Verification items for the finished model (mm, model axes). A direction names the side the tool comes from. Give positions to 0.01 mm unless a question says otherwise; leave off trailing zeros. Loops run counter-clockwise (first coordinate to the right, second up) from the corner with the lowest first, then second, coordinate; pieces in that order, holes last. Notation, with made-up numbers: (26, 42) - (43, 42) arc R17 ccw to (43, 66) - close; hole circle Ø8 at (-5, -22.5). An arc over 180 degrees is marked (long way). Use one line per item in the form item = value.
```python
from build123d import *

# Parameters (mm, degrees)
CROQUIS1_R              = 47.5
SALIENTE_EXTRUIR1_DEPTH = 9
CROQUIS2_R              = 36
SALIENTE_EXTRUIR2_DEPTH = 22
CROQUIS3_R              = 35.5
SALIENTE_EXTRUIR3_DEPTH = 6
CROQUIS4_R              = 35
SALIENTE_EXTRUIR4_DEPTH = 4
CROQUIS5_R              = 34.5
SALIENTE_EXTRUIR5_DEPTH = 4
CROQUIS6_R              = 34
SALIENTE_EXTRUIR6_DEPTH = 24
REDONDEO1_R             = 5
CHAFL_N1_SIZE           = 5.093697795
CHAFL_N1_SIZE_2         = 12
CORTAR_EXTRUIR1_START   = -59.7
CORTAR_EXTRUIR1_DEPTH   = 59.7
MATRIZC1_COUNT          = 8
SALIENTE_EXTRUIR7_REACH = 91.87
CROQUIS8_W              = 0.328373722
CROQUIS8_H              = 2.57874632


with BuildPart() as part:
    # Croquis1 → Saliente-Extruir1 (new body)
    with BuildSketch(Plane.XY):
        Circle(CROQUIS1_R)
    extrude(amount=SALIENTE_EXTRUIR1_DEPTH)

    # Croquis2 → Saliente-Extruir2 (add)
    with BuildSketch(Plane.XY.offset(9)):
        Circle(CROQUIS2_R)
    extrude(amount=SALIENTE_EXTRUIR2_DEPTH)

    # Croquis3 → Saliente-Extruir3 (add)
    with BuildSketch(Plane.XY.offset(31)):
        Circle(CROQUIS3_R)
    extrude(amount=SALIENTE_EXTRUIR3_DEPTH)

    # Croquis4 → Saliente-Extruir4 (add)
    with BuildSketch(Plane.XY.offset(37)):
        Circle(CROQUIS4_R)
    extrude(amount=SALIENTE_EXTRUIR4_DEPTH)

    # Croquis5 → Saliente-Extruir5 (add)
    with BuildSketch(Plane.XY.offset(41)):
        Circle(CROQUIS5_R)
    extrude(amount=SALIENTE_EXTRUIR5_DEPTH)

    # Croquis6 → Saliente-Extruir6 (add)
    with BuildSketch(Plane.XY.offset(45)):
        Circle(CROQUIS6_R)
    extrude(amount=SALIENTE_EXTRUIR6_DEPTH)

    # Redondeo1
    redondeo1_edges = [part.edges().sort_by_distance(p)[0] for p in [
        (-34, 0, 69),
    ]]
    fillet(redondeo1_edges, radius=REDONDEO1_R)

    # Chaflán1
    # the kernel refuses this chamfer: 12, 5.093697795 mm, written as the material it adds along each edge
    with BuildSketch(Plane(origin=(0, 0, 9), x_dir=(1, 0, 0), z_dir=(0, -1, 0))) as chafl_n1_piece_1_section:
        Polygon((36, CHAFL_N1_SIZE), (36 + CHAFL_N1_SIZE_2, 0), (36, 0), align=None)
    chafl_n1_piece_1 = revolve(axis=Axis((0, 0, 9), (0, 0, 1)), mode=Mode.PRIVATE)
    chafl_n1_piece_1 = chafl_n1_piece_1 & Plane(origin=(0, 0, 11.556485036), x_dir=(1, 0, 0), z_dir=(0, 0, -1)) * Cylinder(47.5, 192, mode=Mode.PRIVATE)
    add(chafl_n1_piece_1)

    # Croquis7 → Cortar-Extruir1 (cut)
    with BuildSketch(Plane.XY.offset(69).offset(CORTAR_EXTRUIR1_START)):
        with BuildLine():
            Line((-47.405168495, 3), (-35.624047548, 3))
            ThreePointArc((-35.624047548, 3), (-35.750143548, 0), (-35.624047548, -3))
            Line((-35.624047548, -3), (-47.405168495, -3))
            ThreePointArc((-47.405168495, -3), (-47.5, 0), (-47.405168495, 3))
        make_face()
    cortar_extruir1 = extrude(amount=CORTAR_EXTRUIR1_DEPTH, mode=Mode.SUBTRACT)

    # MatrizC1: Cortar-Extruir1 ×8 about axis
    matrizc1_axis = Axis((0, 0, 0), (0, 0, 1))
    for i in range(1, MATRIZC1_COUNT):
        add(cortar_extruir1.rotate(matrizc1_axis, i * 360 / MATRIZC1_COUNT), mode=Mode.SUBTRACT)

    # Saliente-Extruir7: up to this face of the body (flat: up to its plane)
    saliente_extruir7_end = Plane(part.part.faces().sort_by_distance((0, 0, 0))[0])
    # Croquis8 → Saliente-Extruir7 (add, up to the picked face)
    with BuildSketch(Plane.XY.offset(9.3), mode=Mode.PRIVATE) as saliente_extruir7_sk1:
        with Locations((47.5, 0)):
            Rectangle(CROQUIS8_W, CROQUIS8_H)
    saliente_extruir7_tool1 = split(extrude(saliente_extruir7_sk1.sketch, amount=-SALIENTE_EXTRUIR7_REACH, mode=Mode.PRIVATE), bisect_by=saliente_extruir7_end, keep=Keep.BOTH, mode=Mode.PRIVATE)
    add(saliente_extruir7_tool1.solids().sort_by(Axis((47.5, 0, 9.3), (0, 0, -1)))[0])


solid = part.part
```
1. Section check B-B, the plane x = 0. Record the cut outline in (y, z), then the cut area to 3 significant figures.
Result set:
outline = (-47.5, 0) - (47.5, 0) - (47.5, 9.21) - (47.29, 9.3) - (35.75, 9.3) - (35.75, 31) - (35.5, 31) - (35.5, 37) - (35, 37) - (35, 41) - (34.5, 41) - (34.5, 45) - (34, 45) - (34, 64) arc R5 ccw to (29, 69) - (-29, 69) arc R5 ccw to (-34, 64) - (-34, 45) - (-34.5, 45) - (-34.5, 41) - (-35, 41) - (-35, 37) - (-35.5, 37) - (-35.5, 31) - (-35.75, 31) - (-35.75, 9.3) - (-47.29, 9.3) - (-47.5, 9.21) - close
area = 5,040 mm²
2. Draft check along X on faces 1 (the cylindrical face through (-35.75, 0.04, 20)), 2 (the flat face through (29.26, -25.02, 12.87)), 3 (the flat face through (-41, 0, 9.3)). Enter one of: released by +X, released by -X, zero draft, split by the parting line, or undercut.
Result set:
face_1 = released by -X
face_2 = undercut
face_3 = zero draft
3. Section check D-D, the plane z = 59. Record the cut outline in (x, y), then the cut area to 3 significant figures.
Result set:
outline = circle Ø68 at (0, 0)
area = 3,630 mm²
4. Tool access check on faces 4 (the cylindrical face through (-33.2, 13.92, 22.43)), 5 (the flat face through (-29, 29, 9.3)), 6 (the flat face through (41, 0, 9.3)), 7 (the cylindrical face through (-33.32, -13.63, 22.43)), 8 (the cylindrical face through (13.92, 33.2, 22.43)). Record the directions out of +Z, -Z, +X, -X, +Y, -Y that give a thin tool (end or side, any length) a straight path to the whole face; none if there is none.
Result set:
face_4 = +Z, -X, +Y
face_5 = +Z
face_6 = +Z, +X
face_7 = +Z, -X, -Y
face_8 = +Z, +X, +Y
5. Scan lines: probe 1 along Z at (x, y) = (39.5, -26); probe 2 along Y at (x, z) = (-4, 29.5); probe 3 along X at (y, z) = (-7, 57). Record each from-to range of solid material in increasing order.
Result set:
probe_1 = 0 to 9.3
probe_2 = -35.78 to 35.78
probe_3 = -33.27 to 33.27
6. Depth check by flat-ended pin: pin 1 Ø12.5 at (y, z) = (39.5, 20) entering from +X; pin 2 Ø12 at (y, z) = (-23, 9.5) entering from -X; pin 3 Ø6 at (x, y) = (-30.5, 31.5) entering from +Z; pin 4 Ø10 at (x, y) = (12, 12) entering from -Z. Enter the tip coordinate at first touch or a pass-through.
Result set:
pin_1 = 13.8
pin_2 = -44.35
pin_3 = 11.54
pin_4 = 0
